Model file for the job. Use its own axes, mm. A direction names the side the tool comes from. Coordinates: 2 decimals unless noted, no trailing zeros. Order: outer loops, then holes, each group sorted by start corner. A loop starts at its lowest first (then second) coordinate and runs counter-clockwise, first axis right, second up. Notation, with made-up numbers: (48, 18.5) -> (101, 18.5) arc R21 cw to (101, 56.5) -> close; hole circle Ø2 at (59, 19). An arc over 180 degrees is marked (long way). Use CSV: the item, a comma, the result in double quotes. Start each with the question number.
(1) Pin check, flat tips, straight feed: pin 1 Ø5 at (y, z) = (7.5, 6.5) entering from +X; pin 2 Ø1.5 at (x, z) = (-21.5, 22) entering from +Y; pin 3 Ø6 at (x, z) = (-22.5, 4.5) entering from -Y; pin 4 Ø7 at (x, y) = (-40, 4) entering from +Z. Stop position of each tip, or through.
(2) Cut at B-B on y = 25. Write the cut outline in (x, z), plus the area to 3 significant figures.
(3) Tool access for faces 1 (the flat face through (-28, 29.134, 10)), 2 (the flat face through (0, 18, 22)), 3 (the flat face through (-11, 12, 16.942)), 4 (the flat face through (-44, 4, 8.263)), 5 (the flat face through (-29, 23, 11.989)): list every direction of +Z, -Z, +X, -X, +Y, -Y with a clear straight run to the whole face (end or side of a thin tool).
(4) Cut at D-D on z = 31. Write the cut outline in (x, y), plus the area to 3 significant figures.
(5) Cut at C-C on x = -32. Write the cut outline in (y, z), plus the area to 3 significant figures.
(6) Probe L1, parallel to X at y = 22, z = 21; L2, parallel to Z at x = -49, y = 3.5; L3, parallel to Y at x = -39.5, z = 9.5. List the from-to ranges inside material, lowest first.
(7) Cut at A-A on z = 15. Write the cut outline in (x, y), plus the area to 3 significant figures.
(8) Pull direction X, two halves, no side cores. Call faces 6 (the flat face through (-22, 15, 35.992)), 7 (the flat face through (-20.853, 12, 8)), 8 (the flat face through (-29, 17.087, 24)), 9 (the flat face through (-38.752, 23, 24)): pulls with the +X half, pulls with the -X half, needs draft (parallel to the pull), parting line crosses it, or undercut.
```python
from build123d import *

# Parameters (mm, degrees)
F0_W     = 56.007
F0_H     = 29.1338
F2_DEPTH = 35.9918
F3_W     = 19.9962444603
F3_H     = 12.0468917788
F4_DEPTH = 24.003
F5_W     = 20.8534
F5_H     = 16.9418
F7_DEPTH = 24.003
F8_DEPTH = 8.9916


with BuildPart() as f2:
    # F0 (on Top) → F2 (new body)
    with BuildSketch(Plane.XY):
        with Locations((-28.0035, 14.5669)):
            Rectangle(F0_W, F0_H)
    extrude(amount=F2_DEPTH)

    # F3 (on face) → F4 (cut)
    with BuildSketch(Plane.XY.offset(35.9918)):
        with Locations((-28.7540312856, 23.1103541106)):
            Rectangle(F3_W, F3_H)
    extrude(amount=-F4_DEPTH, mode=Mode.SUBTRACT)

    # F5 (on face) → F7 (cut)
    with BuildSketch(Plane.XZ):
        with Locations((-10.4267, 8.4709)):
            Rectangle(F5_W, F5_H)
    extrude(amount=-F7_DEPTH, mode=Mode.SUBTRACT)

    # F5 (on face) → F8 (cut)
    with BuildSketch(Plane.XZ):
        Polygon((-56.007, 35.9918), (-56.007, 8.2625951707), (-31.0388, 8.2625951707), (-31.0388, 24.003), (-31.0388, 35.9918), align=None)
    extrude(amount=-F8_DEPTH, mode=Mode.SUBTRACT)


solid = f2.part
```
Outcome:
1,pin 1,"x = -20.85"
1,pin 2,"y = 17.09"
1,pin 3,"y = 0"
1,pin 4,"z = 8.26"
2,outline,"(-56.01, 0) -> (0, 0) -> (0, 35.99) -> (-18.76, 35.99) -> (-18.76, 11.99) -> (-38.75, 11.99) -> (-38.75, 35.99) -> (-56.01, 35.99) -> close"
2,area,"1,540 mm2"
3,face 1,"+Z, -Z, +X, -X, +Y"
3,face 2,"+Z, -Z, +X, +Y, -Y"
3,face 3,"-Z, +X, -Y"
3,face 4,"+Z, -X, -Y"
3,face 5,"+Z, +Y"
4,outline,"(-56.01, 8.99) -> (-31.04, 8.99) -> (-31.04, 0) -> (0, 0) -> (0, 29.13) -> (-18.76, 29.13) -> (-18.76, 17.09) -> (-38.75, 17.09) -> (-38.75, 29.13) -> (-56.01, 29.13) -> close"
4,area,"1,170 mm2"
5,outline,"(0, 0) -> (29.13, 0) -> (29.13, 11.99) -> (17.09, 11.99) -> (17.09, 35.99) -> (8.99, 35.99) -> (8.99, 8.26) -> (0, 8.26) -> close"
5,area,"510 mm2"
6,L1,"-56.01 to -38.75, -18.76 to 0"
6,L2,"0 to 8.26"
6,L3,"8.99 to 29.13"
7,outline,"(-56.01, 8.99) -> (-31.04, 8.99) -> (-31.04, 0) -> (-20.85, 0) -> (-20.85, 17.09) -> (-38.75, 17.09) -> (-38.75, 29.13) -> (-56.01, 29.13) -> close; (-18.76, 24) -> (0, 24) -> (0, 29.13) -> (-18.76, 29.13) -> close"
7,area,"680 mm2"
8,face 6,"needs draft"
8,face 7,"pulls with the +X half"
8,face 8,"undercut"
8,face 9,"undercut"
